Check sheet for the modelled part. Datum: model origin and axes. Units: mm. A direction names the side the tool comes from. Round coordinates to 2 decimals unless told otherwise and drop trailing zeros. Order: outer loops, then holes, each group sorted by start corner. A loop starts at its lowest first (then second) coordinate and runs counter-clockwise, first axis right, second up.
Autodesk Fusion 360 part; units mm, degrees
sketch "草图1" plane through (0, 0, 0) normal (0, 0, 1) x (1, 0, 0)
  line L0 (29.8435, -2) -> (-30.1565, -2)
  line L1 (-30.1565, -2) -> (-30.1565, 2)
  line L2 (-30.1565, 2) -> (29.8435, 2)
  line L3 (29.8435, 2) -> (29.8435, -2)
  line L4 (-30.1565, 2) -> (-40.7091, 0)
  line L5 (-40.7091, 0) -> (-30.1565, -2)
  point P0 (-0.1565, 0)
  dimension "d1" = 60
  dimension "d2" = 4
extrude "拉伸1" add sketch "草图1" along normal blind 1.2
sketch "草图2" plane through (0, 0, 0) normal (0, 0, 1) x (1, 0, 0)
  circle A0 centre (9, 0) radius 2.36
  dimension "d5" = 4.72
extrude "拉伸2" add sketch "草图2" along normal blind 12.8
1) Gauge pin test, flat ends, axial feed: pin 1 (1.3 mm diameter, centred on x = -17.5, z = 0.5, fed in from -Y); pin 2 (2 mm diameter, centred on y = -1, z = 8.5, fed in from -X); pin 3 (1.5 mm diameter, centred on y = 0.5, z = 10.5, fed in from +X). Record the tip position at first contact, or that the pin passes through.
2) Sectioned sample at B-B on x = -8. Record the cut outline in (y, z).
3) Sectioned sample at D-D on x = 9.5. Record the cut outline in (y, z), and give its area (3 significant figures).
4) Sectioned sample at A-A on y = -0.7. Record the cut outline in (x, z), and give its area (3 significant figures).
5) Set-up check for faces 1 (the face through (-11, -2, 1)), 2 (the face through (20, 2, 1)), 3 (the face through (20, -2, 1)): record each of +Z, -Z, +X, -X, +Y, -Y from which the full face is reachable in a straight line by a thin tool's end or side.
6) Sectioned sample at C-C on z = 5.25. Record the cut outline in (x, y).
7) Scan lines: line 1 (X direction, y = 0.1, z = 7); line 2 (Z direction, x = -23, y = -0.8); line 3 (X direction, y = 2, z = 4.5). Record each from-to range of solid material in increasing order.
Values found:
1. pin 1: stops at y = -2
1. pin 2: stops at x = 6.64
1. pin 3: stops at x = 11.36
2. outline: (-2, 0) - (2, 0) - (2, 1.2) - (-2, 1.2) - close
3. outline: (-2.31, 0) - (2.31, 0) - (2.31, 12.8) - (-2.31, 12.8) - close
3. area: 59.0 mm2
4. outline: (-37.02, 0) - (29.84, 0) - (29.84, 1.2) - (11.25, 1.2) - (11.25, 12.8) - (6.75, 12.8) - (6.75, 1.2) - (-37.02, 1.2) - close
4. area: 133 mm2
5. face 1: +Z, -Z, -X, -Y
5. face 2: +Z, -Z, +X, +Y
5. face 3: +Z, -Z, +X, -Y
6. outline: circle Ø4.72 at (9, 0)
7. line 1: x = 6.64 to 11.36
7. line 2: z = 0 to 1.2
7. line 3: x = 7.75 to 10.25
